Part model, mm, in its own coordinate system. A direction names the side the tool comes from. Round coordinates to 2 decimals unless told otherwise and drop trailing zeros. Order: outer loops, then holes, each group sorted by start corner. A loop starts at its lowest first (then second) coordinate and runs counter-clockwise, first axis right, second up. Notation, with made-up numbers: (75, 59.25) -> (104, 59.25) arc R29 ccw to (104, 88.25) -> close; hole circle Ø1 at (60, -10.5). An arc over 180 degrees is marked (long way). Answer as a JSON object with one key per item and string values. Group by question number.
```python
from build123d import *

# Parameters (mm, degrees)
F1_DEPTH = 31.75
F3_DEPTH = 12.7
F5_DEPTH = 12.7
F7_DEPTH = 12.7


with BuildPart() as f1:
    # F0 (on Top) → F1 (new body)
    with BuildSketch(Plane.XY):
        Polygon((0, 25.4), (0, 0), (12.7, 0), (12.7, 25.4), (25.4, 25.4), (25.4, 57.15), (-12.7, 57.15), (-12.7, 25.4), align=None)
    extrude(amount=F1_DEPTH)

    # F2 (on face) → F3 (cut)
    with BuildSketch(Plane(origin=(-12.7, 0, 0), x_dir=(0, -1, 0), z_dir=(-1, 0, 0))):
        Polygon((-31.75, 31.75), (-25.4, 0), (-25.4, 31.75), align=None)
    extrude(amount=-F3_DEPTH, mode=Mode.SUBTRACT)

    # F4 (on face) → F5 (cut)
    with BuildSketch(Plane.YZ.offset(25.4)):
        Polygon((25.4, 31.75), (25.4, 0), (31.75, 31.75), align=None)
    extrude(amount=-F5_DEPTH, mode=Mode.SUBTRACT)

    # F6 (on face) → F7 (cut)
    with BuildSketch(Plane.YZ.offset(12.7)):
        Polygon((0, 31.75), (0, 0), (6.35, 31.75), align=None)
    extrude(amount=-F7_DEPTH, mode=Mode.SUBTRACT)


solid = f1.part
```
Q1. Band-saw the part on A-A (z = 16.5). List the corners of the cut face in (x, y), plus the area to 3 significant figures.
Q2. Drop flat-ended pins along their axis: pin 1 Ø3 at (x, z) = (15.5, 8) entering from -Y; pin 2 Ø8 at (x, z) = (11.5, 13.5) entering from -Y. Give the stop position or say it passes through.
Q3. Wall check: line 1 (X direction, y = 12, z = 21); line 2 (Y direction, x = -6, z = 30); line 3 (Y direction, x = 23, z = 16). Give the ranges that are in metal, low to high. Write a range as [from, to].
Q4. Which spindle directions (+Z, -Z, +X, -X, +Y, -Y) get a long thin tool onto all of the face, cutting with end or side? Do faces 1 (the flat face through (25.4, 41, 16)), 2 (the flat face through (0, 16, 16)), 3 (the flat face through (12.7, 16, 16)). Say none if no direction does.
Q5. Band-saw the part on C-C (x = 18). List the corners of the cut face in (y, z).
Q6. Band-saw the part on B-B (y = 28). List the corners of the cut face in (x, z), plus the area to 3 significant figures.
Q7. Band-saw the part on D-D (y = 10). List the corners of the cut face in (x, z).
Completed:
{
 "1": {"outline": "(-12.7, 28.7) -> (0, 28.7) -> (0, 3.3) -> (12.7, 3.3) -> (12.7, 28.7) -> (25.4, 28.7) -> (25.4, 57.15) -> (-12.7, 57.15) -> close", "area": "1,410 mm2"},
 "2": {"pin 1": "y = 26.7", "pin 2": "y = 1.9"},
 "3": {"line 1": "[0, 12.7]", "line 2": "[31.4, 57.15]", "line 3": "[28.6, 57.15]"},
 "4": {"face 1": "+Z, -Z, +X, +Y, -Y", "face 2": "+Z, -X, -Y", "face 3": "+Z, +X, -Y"},
 "5": {"outline": "(25.4, 0) -> (57.15, 0) -> (57.15, 31.75) -> (31.75, 31.75) -> close"},
 "6": {"outline": "(-12.7, 0) -> (25.4, 0) -> (25.4, 13) -> (12.7, 13) -> (12.7, 31.75) -> (0, 31.75) -> (0, 13) -> (-12.7, 13) -> close", "area": "733 mm2"},
 "7": {"outline": "(0, 0) -> (12.7, 0) -> (12.7, 31.75) -> (0, 31.75) -> close"}
}
